```python
from build123d import *

# Parameters (mm, degrees)
SKETCH014_R             = 1.55
SKETCH014_R_2           = 1.5
SKETCH014_R_3           = 3.65
SKETCH014_R_4           = 1.4
SKETCH014_W             = 8
SKETCH014_H             = 3
SKETCH014_W_2           = 12.7
PAD002_DEPTH            = 9.5
POCKET009_DEPTH         = 7
POCKET008_DEPTH         = 10
POCKET010_DEPTH         = 4.5
POCKET013_DEPTH         = 4.5
SKETCH015_W             = 25.7
SKETCH015_H             = 13
POCKET014_DEPTH         = 3
POCKET011_DEPTH         = 2.5
SKETCH013_R             = 1.8
POCKET012_DEPTH         = 1.5
FILLET002_R             = 1
FILLET003_R             = 0.5
BODY002_PLACEMENT_ANGLE = 180


with BuildPart() as part:
    # Sketch014 → Pad002 (new body)
    with BuildSketch(Plane.XY):
        with BuildLine():
            Line((-11, 13.5), (7.5, 13.5))
            ThreePointArc((15.5, 5.5), (13.156854, 11.156854), (7.5, 13.5))
            Line((15.5, 5.5), (15.5, -25.53))
            ThreePointArc((12.7, -28.33), (14.679899, -27.509899), (15.5, -25.53))
            Line((11, -28.33), (12.7, -28.33))
            Line((11, -29.53), (11, -28.33))
            Line((-3, -29.53), (11, -29.53))
            Line((-3, -31.13), (-3, -29.53))
            Line((-3, -31.13), (-16, -31.13))
            Line((-16, -31.13), (-16, 8.5))
            ThreePointArc((-11, 13.5), (-14.535534, 12.035534), (-16, 8.5))
        make_face()
        with Locations((-11, -11)):
            Circle(SKETCH014_R, mode=Mode.SUBTRACT)
        with Locations((11, -11)):
            Circle(SKETCH014_R, mode=Mode.SUBTRACT)
        with Locations((8.5, 8.5)):
            Circle(SKETCH014_R_2, mode=Mode.SUBTRACT)
        with Locations((-10.5, 7)):
            Circle(SKETCH014_R_2, mode=Mode.SUBTRACT)
        with Locations((0.5, 0)):
            Circle(SKETCH014_R_3, mode=Mode.SUBTRACT)
        with Locations((-5.5, 8.5)):
            Circle(SKETCH014_R_4, mode=Mode.SUBTRACT)
        with Locations((-8.7, -25.79)):
            Rectangle(SKETCH014_W, SKETCH014_H, mode=Mode.SUBTRACT)
        with Locations((6.35, -25.79)):
            Rectangle(SKETCH014_W_2, SKETCH014_H, mode=Mode.SUBTRACT)
    extrude(amount=PAD002_DEPTH)

    # Sketch012 (on Face27 of Pad002) → Pocket009 (cut)
    with BuildSketch(Plane.XY.offset(9.5)):
        with BuildLine():
            Line((7.85, -4), (7.75, -4))
            ThreePointArc((7.75, -4), (7.042893, -4.292893), (6.75, -5))
            Line((6.75, -5), (6.75, -5.35))
            ThreePointArc((5.85, -6.25), (6.486396, -5.986396), (6.75, -5.35))
            Line((5.85, -6.25), (-4.85, -6.25))
            ThreePointArc((-5.75, -5.35), (-5.486396, -5.986396), (-4.85, -6.25))
            Line((-5.75, -5.35), (-5.75, -5))
            ThreePointArc((-5.75, -5), (-6.042893, -4.292893), (-6.75, -4))
            Line((-6.75, -4), (-6.85, -4))
            ThreePointArc((-7.75, -3.1), (-7.486396, -3.736396), (-6.85, -4))
            Line((-7.75, -3.1), (-7.75, 3.1))
            ThreePointArc((-6.85, 4), (-7.486396, 3.736396), (-7.75, 3.1))
            Line((-6.85, 4), (-6.75, 4))
            ThreePointArc((-6.75, 4), (-6.042893, 4.292893), (-5.75, 5))
            Line((-5.75, 5), (-5.75, 5.35))
            ThreePointArc((-4.85, 6.25), (-5.486396, 5.986396), (-5.75, 5.35))
            Line((-4.85, 6.25), (5.85, 6.25))
            ThreePointArc((6.75, 5.35), (6.486396, 5.986396), (5.85, 6.25))
            Line((6.75, 5.35), (6.75, 5))
            ThreePointArc((6.75, 5), (7.042893, 4.292893), (7.75, 4))
            Line((7.75, 4), (7.85, 4))
            ThreePointArc((8.75, 3.1), (8.486396, 3.736396), (7.85, 4))
            Line((8.75, 3.1), (8.75, -3.1))
            ThreePointArc((7.85, -4), (8.486396, -3.736396), (8.75, -3.1))
        make_face()
    extrude(amount=-POCKET009_DEPTH, mode=Mode.SUBTRACT)

    # Sketch016 (on Face5 of Pocket009) → Pocket008 (cut)
    with BuildSketch(Plane.XY.offset(9.5)):
        with BuildLine():
            Line((12.75, 7), (16.5, 7))
            Line((16.5, 7), (16.5, -7))
            Line((16.5, -7), (12.75, -7))
            ThreePointArc((11.5, -5.75), (11.866117, -6.633883), (12.75, -7))
            Line((11.5, -5.75), (11.5, 5.75))
            ThreePointArc((12.75, 7), (11.866117, 6.633883), (11.5, 5.75))
        make_face()
    extrude(amount=-POCKET008_DEPTH, mode=Mode.SUBTRACT)

    # Sketch017 (on Face5 of Pocket008) → Pocket010 (cut)
    with BuildSketch(Plane.XY.offset(9.5)):
        Polygon((-8.1, -12.674316), (-8.1, -9.325684), (-11, -7.651368), (-13.9, -9.325684), (-13.9, -12.674316), (-11, -14.348632), align=None)
        Polygon((13.9, -12.674316), (13.9, -9.325684), (11, -7.651368), (8.1, -9.325684), (8.1, -12.674316), (11, -14.348632), align=None)
    extrude(amount=-POCKET010_DEPTH, mode=Mode.SUBTRACT)

    # Sketch018 (on Face5 of Pocket010) → Pocket013 (cut)
    with BuildSketch(Plane.XY.offset(9.5)):
        Polygon((-7.85, 5.470022), (-7.85, 8.529978), (-10.5, 10.059956), (-13.15, 8.529978), (-13.15, 5.470022), (-10.5, 3.940044), align=None)
    extrude(amount=-POCKET013_DEPTH, mode=Mode.SUBTRACT)

    # Sketch015 (on Face4 of Pocket013) → Pocket014 (cut)
    with BuildSketch(Plane(origin=(0, 0, 0), x_dir=(1, 0, 0), z_dir=(0, 0, -1))):
        with Locations((0, 22)):
            Rectangle(SKETCH015_W, SKETCH015_H)
    extrude(amount=-POCKET014_DEPTH, mode=Mode.SUBTRACT)

    # Sketch019 → Pocket011 (cut)
    with BuildSketch(Plane(origin=(0, 0, 0), x_dir=(1, 0, 0), z_dir=(0, 0, -1))):
        with BuildLine():
            Line((-16, -10), (-11, -10))
            ThreePointArc((-10, -11), (-10.292893, -10.292893), (-11, -10))
            Line((-10, -11), (-10, -14))
            Line((-10, -14), (-16, -14))
            Line((-16, -14), (-16, -10))
        make_face()
    extrude(amount=-POCKET011_DEPTH, mode=Mode.SUBTRACT)

    # Sketch013 (on Face83 of Pocket011) → Pocket012 (cut)
    with BuildSketch(Plane(origin=(0, 0, 3), x_dir=(1, 0, 0), z_dir=(0, 0, -1))):
        with Locations((0, 22)):
            Circle(SKETCH013_R)
        with BuildLine():
            Line((-12.85, 20.5), (-3.5, 20.5))
            ThreePointArc((-1.5, 18.5), (-2.085786, 19.914214), (-3.5, 20.5))
            Line((-1.5, 18.5), (-1.5, 15.5))
            Line((-1.5, 15.5), (-12.85, 15.5))
            Line((-12.85, 15.5), (-12.85, 20.5))
        make_face()
        with BuildLine():
            Line((1.5, 15.5), (12.85, 15.5))
            Line((12.85, 15.5), (12.85, 20.5))
            Line((12.85, 20.5), (3.5, 20.5))
            ThreePointArc((3.5, 20.5), (2.085786, 19.914214), (1.5, 18.5))
            Line((1.5, 18.5), (1.5, 15.5))
        make_face()
        with BuildLine():
            Line((-12.85, 23.5), (-3.5, 23.5))
            ThreePointArc((-3.5, 23.5), (-2.085786, 24.085786), (-1.5, 25.5))
            Line((-1.5, 25.5), (-1.5, 28.5))
            Line((-1.5, 28.5), (-12.85, 28.5))
            Line((-12.85, 28.5), (-12.85, 23.5))
        make_face()
        with BuildLine():
            Line((1.5, 28.5), (12.85, 28.5))
            Line((12.85, 28.5), (12.85, 23.5))
            Line((12.85, 23.5), (3.5, 23.5))
            ThreePointArc((1.5, 25.5), (2.085786, 24.085786), (3.5, 23.5))
            Line((1.5, 25.5), (1.5, 28.5))
        make_face()
    extrude(amount=-POCKET012_DEPTH, mode=Mode.SUBTRACT)

    # Fillet002
    fillet002_edges = [part.edges().sort_by_distance(p)[0] for p in [
        (15.358117, 7, 4.75),
        (15.5, -7, 4.75),
        (11, -29.53, 4.75),
        (-3, -31.13, 4.75),
        (-16, -31.13, 4.75),
        (-15.769696, 10, 1.25),
        (-10, 13.5, 1.25),
    ]]
    fillet(fillet002_edges, radius=FILLET002_R)

    # Fillet003
    fillet003_edges = [part.edges().sort_by_distance(p)[0] for p in [
        (-3, -29.53, 4.75),
        (-12.85, -15.5, 1.5),
        (-12.85, -15.5, 3.75),
        (1.5, -15.5, 3.75),
        (-12.85, -23.5, 3.75),
        (-12.85, -28.5, 3.75),
        (-12.85, -28.5, 1.5),
        (-12.85, -20.5, 3.75),
        (-12.7, -27.29, 7),
        (-1.5, -15.5, 3.75),
        (-4.7, -24.29, 7),
        (-4.7, -27.29, 7),
        (-12.7, -24.29, 7),
        (-1.5, -28.5, 3.75),
        (1.5, -28.5, 3.75),
        (1.5, -27.29, 3.75),
        (0, -27.29, 6.25),
        (0, -24.29, 6.25),
        (1.907549, -24.29, 3.75),
        (12.85, -20.5, 3.75),
        (12.7, -27.29, 7),
        (12.85, -23.5, 3.75),
        (12.85, -15.5, 3.75),
        (12.85, -15.5, 1.5),
        (12.7, -24.29, 7),
        (-1.8, -22, 4.5),
    ]]
    fillet(fillet003_edges, radius=FILLET003_R)


with BuildPart() as part_1:
    # Body002 placement: moved
    add(part.part.moved(Location((-62, 35, 110))).rotate(Axis((-62, 35, 110), (0, 1, 0)), BODY002_PLACEMENT_ANGLE))


solid = part_1.part
```
The listing builds one solid part. Answer for the finished solid, in the listing's coordinates (mm). A direction names the side the tool comes from. Round coordinates to 2 decimals unless told otherwise and drop trailing zeros. Loops run counter-clockwise (first coordinate to the right, second up) from the corner with the lowest first, then second, coordinate; pieces in that order, holes last. Notation, with made-up numbers: (-11.5, 14) - (18.5, 14) arc R27 cw to (18.5, 44) - close; hole circle Ø10 at (-35.75, -2). An arc over 180 degrees is marked (long way). Use one line per item in the form item = value. Start each with the question number.
1. For a pull along X with two mould halves and no side action, classify faces 5 (the face through (-70.75, 35, 104)), 6 (the face through (-76.854, 42.422, 105.317)), 7 (the face through (-53, 3.87, 105)) as pulls with the +X half, pulls with the -X half, needs draft (parallel to the pull), parting line crosses it, or undercut.
2. The part is cut by section B-B on y = 13. Determine the outline of the cut face in (x, z), then the cut area to 3 significant figures.
3. The part is cut by section C-C on z = 108.75. Give the number of separate pieces and of enclosed holes in the cut face, then the cut area to 3 significant figures.
4. Consider line 1 (X direction, y = 14, z = 106.75); line 2 (Y direction, x = -70, z = 103); line 3 (Y direction, x = -51, z = 108.05). Determine where each line is inside the solid, lowest interval first. Write a range as [from, to].
5. The part is cut by section A-A on y = 35. Determine the outline of the cut face in (x, z).
6. Given pin 1 Ø1.7 at (x, y) = (-56.5, 43.5) entering from +Z; pin 2 Ø3.5 at (x, z) = (-61.5, 107) entering from -Y; pin 3 Ø1.4 at (x, z) = (-75, 103) entering from +Y, each flat-ended and moving along its own axis, determine where each tip first touches the part or whether it passes through.
7. A tool of negligible diameter and unlimited length cuts with its end or side. For faces 1 (the face through (-74.43, 21.477, 102.718)), 2 (the face through (-74, 6.67, 103)), 3 (the face through (-60, 13, 107)), 4 (the face through (-68, 7.71, 103)), from which of +Z, -Z, +X, -X, +Y, -Y can it reach the whole face along a straight path? Write none if from no direction.
Geometry check:
q1.face_5 = undercut
q1.face_6 = pulls with the -X half
q1.face_7 = needs draft
q2.outline = (-77.5, 100.5) - (-46, 100.5) - (-46, 110) - (-49.15, 110) - (-49.15, 107) - (-60.2, 107) - (-60.2, 106) arc R0.5 cw to (-60.7, 105.5) - (-63.3, 105.5) arc R0.5 cw to (-63.8, 106) - (-63.8, 107) - (-74.85, 107) - (-74.85, 110) - (-77.5, 110) - close
q2.area = 217 mm^2
q3.separate_pieces = 1
q3.enclosed_holes = 6
q3.area = 867 mm^2
q4.line_1 = [-77.5, -63.5], [-60.5, -46]
q4.line_2 = [5.47, 7.71], [10.71, 31.01], [38.99, 42.09], [44.91, 48.48]
q4.line_3 = [3.87, 6.5], [19.5, 22.45], [25.55, 40.59], [43.41, 45]
q5.outline = (-73.5, 100.5) - (-70.75, 100.5) - (-70.75, 107.5) - (-66.15, 107.5) - (-66.15, 110) - (-73.5, 110) - close; (-58.85, 107.5) - (-54.25, 107.5) - (-54.25, 100.5) - (-46, 100.5) - (-46, 110) - (-58.85, 110) - close
q6.pin_1 = through
q6.pin_2 = 5.47
q6.pin_3 = 46.9
q7.face_1 = -Z
q7.face_2 = +Z, -Z, -X, -Y
q7.face_3 = +Z
q7.face_4 = +Z, -Z
